Can you work these out from the drawing? Everything is in mm from the part's minimum corner. Coordinates: 2 decimals unless noted, no trailing zeros. Order: outer loops, then holes, each group sorted by start corner. A loop starts at its lowest first (then second) coordinate and runs counter-clockwise, first axis right, second up. Notation, with made-up numbers: (26, 85.5) -> (37, 85.5) arc R14 ccw to (37, 93.5) -> close; hole circle Ø5 at (7.25, 17). An arc over 180 degrees is marked (long way). Return JSON: item names as keys, results as strings. Group by question number.
1) If we section it at C-C, the plane y = 271.5: Please give me the cut outline in (x, z), then the cut area to 3 significant figures.
2) If we section it at B-B, the plane x = 20: Please give me the cut outline in (y, z), then the cut area to 3 significant figures.
3) If I drill on probe 1 along Y at (x, z) = (31, 31.5); probe 2 along Y at (x, z) = (36.5, 31); probe 3 along Z at (x, y) = (9.5, 256), over which ranges is the centre line in solid material (lowest first)? Write a range as from..to.
4) For pin 1 (2 mm diameter, centred on y = 173.5, z = 38.5, fed in from -X), with a flat end and sliding along its axis, tell me the tip position at first contact or that it passes through.
5) If we section it at A-A, the plane z = 34.5: Please give me the cut outline in (x, y), then the cut area to 3 significant figures.
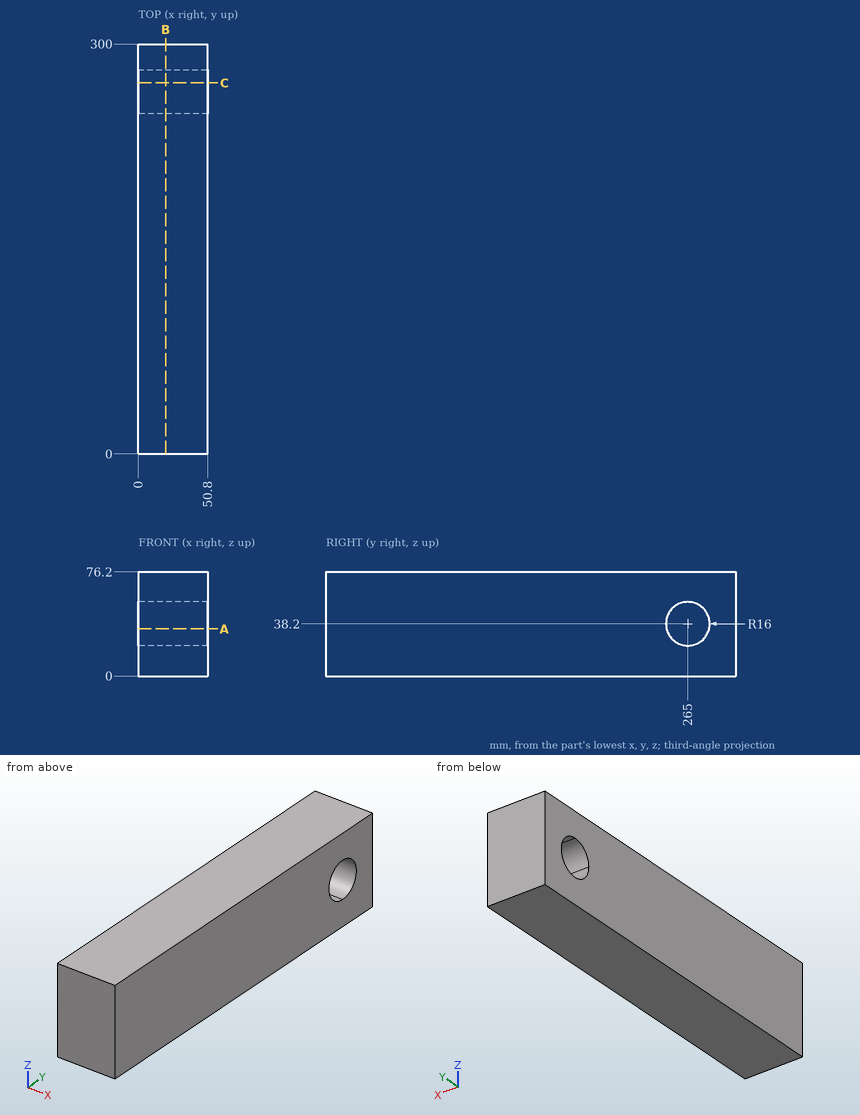
Result sheet:
{
 "1": {"outline": "(0, 0) -> (50.8, 0) -> (50.8, 23.58) -> (0, 23.58) -> close; (0, 52.82) -> (50.8, 52.82) -> (50.8, 76.2) -> (0, 76.2) -> close", "area": "2,390 mm2"},
 "2": {"outline": "(0, 0) -> (300, 0) -> (300, 76.2) -> (0, 76.2) -> close; hole circle Ø32 at (265, 38.2)", "area": "22,100 mm2"},
 "3": {"probe 1": "y = 0..250.47, 279.53..300", "probe 2": "y = 0..250.71, 279.29..300", "probe 3": "z = 0..24.97, 51.43..76.2"},
 "4": {"pin 1": "stops at x = 0"},
 "5": {"outline": "(0, 0) -> (50.8, 0) -> (50.8, 249.43) -> (0, 249.43) -> close; (0, 280.57) -> (50.8, 280.57) -> (50.8, 300) -> (0, 300) -> close", "area": "13,700 mm2"}
}
